Verification items for the finished model (mm, model axes). A direction names the side the tool comes from. Round coordinates to 2 decimals unless told otherwise and drop trailing zeros. Write each loop counter-clockwise with the first axis right and the second up, starting at its lowest first coordinate (ties: lowest second). Pieces come first, ordered by that corner, then holes. Notation, with made-up numbers: (51, -37) - (76, -37) arc R20 cw to (76, -32) - close; hole circle Ø2 at (-18, 44.25). An arc over 180 degrees is marked (long way). Answer as a JSON object with one key per item and string values.
```python
from build123d import *

# Parameters (mm, degrees)
BASE_FLANGE1_DEPTH        = 3
SKETCH8_R                 = 1.635
CUT_EXTRUDE1_DEPTH        = 3
F_4_CLEARANCE_HOLE2_D     = 3.2639
F_4_CLEARANCE_HOLE2_DEPTH = 3
F_4_CLEARANCE_HOLE2_TIP   = 0.980574487
CUT_EXTRUDE2_DEPTH        = 3


# Sheet-metal steps are written as plain solids
with BuildPart() as part:
    # Sketch3 → Base-Flange1 (new body)
    with BuildSketch(Plane(origin=(0, 0, 0), x_dir=(1, 0, 0), z_dir=(0, 1, 0))):
        with BuildLine():
            Line((-29.358964924, 8.867320879), (-29.358964924, 25.825))
            Line((-29.358964924, 25.825), (-29.358964924, 48.325))
            Line((-29.358964924, 48.325), (-19.358964924, 48.325))
            Line((-19.358964924, 48.325), (-19.358964924, 25.825))
            Line((-19.358964924, 25.825), (29.358964924, 25.825))
            Line((29.358964924, 25.825), (29.358964924, 8.867320879))
            ThreePointArc((29.358964924, 8.867320879), (23.15, 10.825), (16.941035076, 8.867320879))
            ThreePointArc((16.941035076, 8.867320879), (11.575, 6.362392354), (6.208964924, 8.867320879))
            ThreePointArc((6.208964924, 8.867320879), (0, 10.825), (-6.208964924, 8.867320879))
            ThreePointArc((-6.208964924, 8.867320879), (-11.575, 6.362392354), (-16.941035076, 8.867320879))
            ThreePointArc((-16.941035076, 8.867320879), (-23.15, 10.825), (-29.358964924, 8.867320879))
        make_face()
    extrude(amount=-BASE_FLANGE1_DEPTH)

    # Sketch8 → Cut-Extrude1 (cut)
    with BuildSketch(Plane(origin=(0, 0, 0), x_dir=(1, 0, 0), z_dir=(0, 1, 0))):
        with Locations(Location((-24.358964924, 44.325, 0), (0, 0, 270))):
            Circle(SKETCH8_R)
        with Locations(Location((-24.358964924, 34.825, 0), (0, 0, 270))):
            Circle(SKETCH8_R)
    extrude(amount=-CUT_EXTRUDE1_DEPTH, mode=Mode.SUBTRACT)

    # #4 Clearance Hole2
    with Locations(Plane.XZ.offset(3)):
        with Locations((11.575, -18.325), (-11.575, -18.325)):
            Hole(F_4_CLEARANCE_HOLE2_D / 2, depth=F_4_CLEARANCE_HOLE2_DEPTH)
            with Locations((0, 0, -(F_4_CLEARANCE_HOLE2_DEPTH + F_4_CLEARANCE_HOLE2_TIP / 2))):  # 118° drill point
                Cone(0, F_4_CLEARANCE_HOLE2_D / 2, F_4_CLEARANCE_HOLE2_TIP, mode=Mode.SUBTRACT)

    # Sketch11 → Cut-Extrude2 (cut)
    with BuildSketch(Plane.XZ.offset(3)):
        with BuildLine():
            Line((-29.645753142, -9.276896902), (-29.645753142, -3.891418545))
            Line((-29.645753142, -3.891418545), (33.433786827, -3.891418545))
            Line((33.433786827, -3.891418545), (33.433786827, -25.825))
            Line((33.433786827, -25.825), (28.858964924, -25.825))
            Line((28.858964924, -25.825), (28.858964924, -9.780764004))
            ThreePointArc((28.858964924, -9.780764004), (22.648874034, -11.313907272), (16.598650974, -9.237718925))
            ThreePointArc((16.598650974, -9.237718925), (11.575, -6.862392354), (6.551349026, -9.237718925))
            ThreePointArc((6.551349026, -9.237718925), (0, -11.325), (-6.551349026, -9.237718925))
            ThreePointArc((-6.551349026, -9.237718925), (-11.575, -6.862392354), (-16.598650974, -9.237718925))
            ThreePointArc((-16.598650974, -9.237718925), (-23.115993323, -11.324948942), (-29.645753142, -9.276896902))
        make_face()
    extrude(amount=-CUT_EXTRUDE2_DEPTH, mode=Mode.SUBTRACT)


solid = part.part
```
Q1. Material ranges on line 1 along X through (y, z) = (-0.8, -10); line 2 along X through (y, z) = (-2.1, -19.5); line 3 along X through (y, z) = (-0.85, -19), recorded low to high. Write a range as [from, to].
Geometry check:
{"line 1": "x = [-29.36, -28.47], [-17.83, -5.32], [5.32, 17.83], [28.47, 28.86]", "line 2": "x = [-29.36, -12.71], [-10.44, 10.44], [12.71, 28.86]", "line 3": "x = [-29.36, -13.06], [-10.09, 10.09], [13.06, 28.86]"}
Q2. Section check B-B, the plane y = -0.45. Record the cut outline in (x, z) (3 decimals), then the cut area to 3 significant figures.
Geometry check:
{"outline": "(-29.359, -48.325) - (-19.359, -48.325) - (-19.359, -25.825) - (28.859, -25.825) - (28.859, -9.781) arc R11.325 cw to (16.599, -9.238) arc R6.5 ccw to (6.551, -9.238) arc R11.325 cw to (-6.551, -9.238) arc R6.5 ccw to (-16.599, -9.238) arc R11.325 cw to (-29.359, -9.471) - close; hole circle Ø3.27 at (-24.359, -44.325); hole circle Ø3.27 at (-24.359, -34.825); hole circle Ø3.264 at (-11.575, -18.325); hole circle Ø3.264 at (11.575, -18.325)", "area": "1,130 mm2"}
Q3. Section check D-D, the plane x = 23.5. Record the cut outline in (y, z) (3 decimals), then the cut area to 3 significant figures.
Geometry check:
{"outline": "(-3, -25.825) - (0, -25.825) - (0, -11.32) - (-3, -11.32) - close", "area": "43.5 mm2"}
Q4. Release check for a two-part mould opening along X. For faces 3 (the flat face through (4, -1, -25.825)), 4 (the flat face through (-29.359, -1, -29)), 5 (the cylindrical face through (22.74, -1.521, -11.318)) record: released by +X, released by -X, zero draft, split by the parting line, or undercut.
Geometry check:
{"face 3": "zero draft", "face 4": "released by -X", "face 5": "undercut"}
Q5. Set-up check for faces 1 (the flat face through (-19.359, -1, -37)), 2 (the flat face through (-24, -1, -48.325)): record each of +Z, -Z, +X, -X, +Y, -Y from which the full face is reachable in a straight line by a thin tool's end or side.
Geometry check:
{"face 1": "-Z, +X, +Y, -Y", "face 2": "-Z, +X, -X, +Y, -Y"}
Q6. Section check A-A, the plane z = -45. Record the cut outline in (x, y), then the cut area to 3 significant figures.
Geometry check:
{"outline": "(-29.36, -3) - (-25.85, -3) - (-25.85, 0) - (-29.36, 0) - close; (-22.87, -3) - (-19.36, -3) - (-19.36, 0) - (-22.87, 0) - close", "area": "21.1 mm2"}
Q7. Section check C-C, the plane x = 1.5. Record the cut outline in (y, z) (3 decimals).
Geometry check:
{"outline": "(-3, -25.825) - (0, -25.825) - (0, -11.225) - (-3, -11.225) - close"}
Q8. Gauge pin test, flat ends, axial feed: P1, Ø2, axis at x = -24.36, z = -44.32, coming from the +Y side; P2, Ø0.9, axis at y = -1, z = -34, coming from the +X side. Record the tip position at first contact, or that the pin passes through.
Geometry check:
{"P1": "passes through", "P2": "stops at x = -19.36"}
